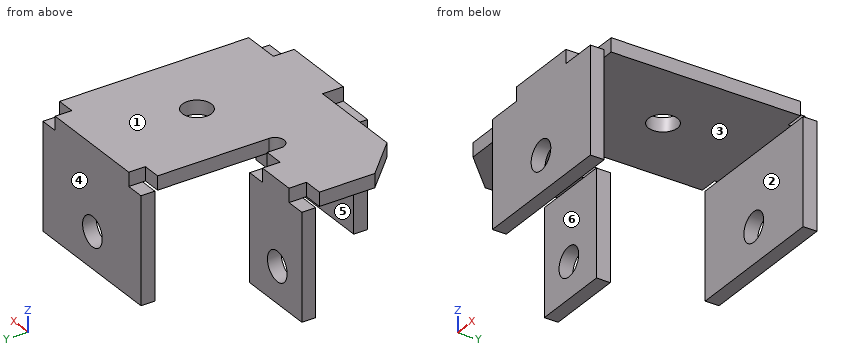
from build123d import *

# Parameters (mm, degrees)
SKETCH1_R           = 1.575
BOSS_EXTRUDE1_DEPTH = 1.5
SKETCH2_W           = 15.95
SKETCH2_H           = 1.5
SKETCH2_W_2         = 8.5
BOSS_EXTRUDE2_DEPTH = 11.5
SKETCH3_R           = 1.6
CUT_EXTRUDE1_DEPTH  = 38.875519798


with BuildPart() as part:
    # Sketch1 → Boss-Extrude1 (new body)
    with BuildSketch(Plane.XY):
        with BuildLine():
            Line((0, -10.25), (0, 10.25))
            Line((0, 10.25), (-1.975, 10.25))
            Line((-1.975, 10.25), (-1.975, 12.05))
            Line((-1.975, 12.05), (-13.975, 12.05))
            Line((-13.975, 12.05), (-13.975, 10.25))
            Line((-13.975, 10.25), (-15.95, 10.25))
            Line((-15.95, 10.25), (-15.95, -1.8))
            ThreePointArc((-15.95, -1.8), (-16.95, -2.8), (-17.95, -1.8))
            Line((-17.95, -1.8), (-17.95, -0.3))
            Line((-17.95, -0.3), (-20.05, -0.3))
            Line((-20.05, -0.3), (-20.05, 1.6))
            Line((-20.05, 1.6), (-24.35, 1.6))
            Line((-24.35, 1.6), (-24.35, -0.3))
            Line((-24.35, -0.3), (-26.45, -0.3))
            Line((-26.45, -0.3), (-26.45, -6.3))
            Line((-26.45, -6.3), (-22.5, -10.25))
            Line((-22.5, -10.25), (-12, -10.25))
            Line((-12, -10.25), (-12, -12.5))
            Line((-12, -12.5), (-4, -12.5))
            Line((-4, -12.5), (-4, -10.25))
            Line((-4, -10.25), (0, -10.25))
        make_face()
        with Locations((-7.975, 0.675)):
            Circle(SKETCH1_R, mode=Mode.SUBTRACT)
    extrude(amount=BOSS_EXTRUDE1_DEPTH)

    # Sketch2 → Boss-Extrude2 (add)
    with BuildSketch(Plane(origin=(0, 0, 0), x_dir=(-1, 0, 0), z_dir=(0, 0, -1))):
        with Locations((7.975, 11.3)):
            Rectangle(SKETCH2_W, SKETCH2_H)
        with Locations((7.975, -11.75)):
            Rectangle(SKETCH2_W, SKETCH2_H)
        with Locations((22.2, 0.85)):
            Rectangle(SKETCH2_W_2, SKETCH2_H)
    extrude(amount=BOSS_EXTRUDE2_DEPTH)

    # Sketch3 → Cut-Extrude1 (cut, through all)
    with BuildSketch(Plane(origin=(0, 12.05, 0), x_dir=(1, 0, 0), z_dir=(0, 1, 0))):
        with Locations(Location((-8.05, 7.6, 0), (0, 0, 270))):
            Circle(SKETCH3_R)
        with Locations(Location((-22.45, 7.6, 0), (0, 0, 270))):
            Circle(SKETCH3_R)
    extrude(amount=-CUT_EXTRUDE1_DEPTH, mode=Mode.SUBTRACT)


solid = part.part
For this review, take the finished solid that the model builds, in its own axes (mm). Face numbers are marked on the shaded views. A direction names the side the tool comes from. Give positions to 0.01 mm unless a question says otherwise; leave off trailing zeros. Order: outer loops, then holes, each group sorted by start corner. A loop starts at its lowest first (then second) coordinate and runs counter-clockwise, first axis right, second up. Notation, with made-up numbers: M -30.75,64 L 5.25,64 A10 ccw 5.25,70 Z; hole C 40,7.25 d10. An arc over 180 degrees is marked long. Answer in a Markdown table with one row per item. Add a question column.
(1) Consider section B-B on x = -2.5. State the section outline as (y, z) points.
(2) Consider section A-A on z = -7.6. State the section outline as (x, y) points, and give its area (3 significant figures).
(3) Mouldability with a two-part tool opening along Y and no side actions: class the marked faces 3, 4, 5 and 6 as +Y half, -Y half, draft (parallel to the pull), parting line (faces both ways), or undercut.
(4) Wall thickness on probe 1 along Y at (x, z) = (-13, -7); probe 2 along X at (y, z) = (-0.75, 0.5); probe 3 along Z at (x, y) = (-6, -2.75): over which ranges is each line inside the solid? List them lowest first. Write a range as [from, to].
(5) Consider section D-D on x = -6. State the section outline as (y, z) points, and give its area (3 significant figures).
(6) Consider section C-C on z = -10.25. State the section outline as (x, y) points, and give its area (3 significant figures).
(7) For the marked faces 1 and 2, list the 3-axis set-ups (+Z, -Z, +X, -X, +Y, -Y) from which the entire face can be reached by the end or side of a thin tool; tool diameter is ignored.
(8) For pin 1 (0.8 mm diameter, centred on x = -19.5, z = 0.5, fed in from +Y); pin 2 (1.5 mm diameter, centred on x = -11, y = 9, fed in from -Z); pin 3 (0.8 mm diameter, centred on x = -14, y = -11.5, fed in from +Z), all flat-tipped, find the tip position at first contact; note any pin that passes through.
Evaluation:
| question | item | result |
|---|---|---|
| 1 | outline | M -12.5,-11.5 L -11,-11.5 L -11,0 L -12.5,0 Z; M -10.25,0 L 10.55,0 L 10.55,-11.5 L 12.05,-11.5 L 12.05,1.5 L -10.25,1.5 Z |
| 2 | outline | M -26.45,0.1 L -24.05,0.1 L -24.05,1.6 L -26.45,1.6 Z; M -20.85,0.1 L -17.95,0.1 L -17.95,1.6 L -20.85,1.6 Z; M -15.95,-12.5 L -9.65,-12.5 L -9.65,-11 L -15.95,-11 Z; M -15.95,10.55 L -9.65,10.55 L -9.65,12.05 L -15.95,12.05 Z; M -6.45,-12.5 L 0,-12.5 L 0,-11 L -6.45,-11 Z; M -6.45,10.55 L 0,10.55 L 0,12.05 L -6.45,12.05 Z |
| 2 | area | 46.2 mm^2 |
| 3 | face 3 | undercut |
| 3 | face 4 | +Y half |
| 3 | face 5 | undercut |
| 3 | face 6 | -Y half |
| 4 | probe 1 | y = [-12.5, -11], [10.55, 12.05] |
| 4 | probe 2 | x = [-26.45, -17.95], [-15.95, -8.65], [-7.3, 0] |
| 4 | probe 3 | z = [0, 1.5] |
| 5 | outline | M -12.5,-11.5 L -11,-11.5 L -11,0 L 10.55,0 L 10.55,-11.5 L 12.05,-11.5 L 12.05,1.5 L -12.5,1.5 Z |
| 5 | area | 71.3 mm^2 |
| 6 | outline | M -26.45,0.1 L -17.95,0.1 L -17.95,1.6 L -26.45,1.6 Z; M -15.95,-12.5 L 0,-12.5 L 0,-11 L -15.95,-11 Z; M -15.95,10.55 L 0,10.55 L 0,12.05 L -15.95,12.05 Z |
| 6 | area | 60.6 mm^2 |
| 7 | face 1 | +Z, +X, -X, +Y, -Y |
| 7 | face 2 | -Z, +X, -X |
| 8 | pin 1 | stops at y = -0.3 |
| 8 | pin 2 | stops at z = 0 |
| 8 | pin 3 | stops at z = 0 |
